Build history of the part. All positions in model axes, mm. A direction names the side the tool comes from. Give positions to 0.01 mm unless a question says otherwise; leave off trailing zeros. Order: outer loops, then holes, each group sorted by start corner. A loop starts at its lowest first (then second) coordinate and runs counter-clockwise, first axis right, second up. Notation, with made-up numbers: (2.25, 50) - (6.25, 50) arc R17 cw to (6.25, 82) - close; hole circle Ø4 at (34, 73). An arc over 180 degrees is marked (long way). Use a Markdown table: item, result.
from build123d import *

# Parameters (mm, degrees)
F0_W     = 3.175
F0_H     = 66.04
F1_DEPTH = 3.175
F2_DEPTH = 66.04
F3_R     = 5.08
F4_W     = 70.348228
F4_H     = 17.78
F5_DEPTH = 3.175
F4_R     = 5.08
F4_R_2   = 3.556
F6_DEPTH = 25.4
F7_R     = 0.508


with BuildPart() as f1:
    # F0 (on Top) → F1 (new body)
    with BuildSketch(Plane.XY):
        with Locations((42.8625, 0)):
            Rectangle(F0_W, F0_H)
        with Locations((-42.8625, 0)):
            Rectangle(F0_W, F0_H)
        with BuildLine():
            Line((41.275, -33.02), (41.275, 33.02))
            Line((41.275, 33.02), (3.81, 33.02))
            ThreePointArc((3.81, 33.02), (0, 29.21), (-3.81, 33.02))
            Line((-3.81, 33.02), (-41.275, 33.02))
            Line((-41.275, 33.02), (-41.275, -33.02))
            Line((-41.275, -33.02), (41.275, -33.02))
        make_face()
    extrude(amount=F1_DEPTH)

    # F0 (on Top) → F2 (join)
    with BuildSketch(Plane.XY):
        with Locations((-42.8625, 0)):
            Rectangle(F0_W, F0_H)
        with Locations((42.8625, 0)):
            Rectangle(F0_W, F0_H)
    extrude(amount=-F2_DEPTH)

    # F3
    f3_edges = [f1.edges().sort_by_distance(p)[0] for p in [
        (-44.45, 0, 3.175),
        (44.45, 0, 3.175),
    ]]
    fillet(f3_edges, radius=F3_R)

    # F4 (on face) → F5 (join)
    with BuildSketch(Plane(origin=(0, 0, 0), x_dir=(1, 0, 0), z_dir=(0, 0, -1))):
        Rectangle(F4_W, F4_H)
        Polygon((-18.800886, 0), (-22.100443, -5.715), (-28.699557, -5.715), (-31.999114, 0), (-28.699557, 5.715), (-22.100443, 5.715), align=None, mode=Mode.SUBTRACT)
        Polygon((30.23935, 0), (27.819675, -4.191), (22.980325, -4.191), (20.56065, 0), (22.980325, 4.191), (27.819675, 4.191), align=None, mode=Mode.SUBTRACT)
    extrude(amount=F5_DEPTH)

    # F4 (on face) → F6 (cut)
    with BuildSketch(Plane(origin=(0, 0, 0), x_dir=(1, 0, 0), z_dir=(0, 0, -1))):
        with Locations((-25.4, 0)):
            Circle(F4_R)
        with Locations((25.4, 0)):
            Circle(F4_R_2)
    extrude(amount=-F6_DEPTH, mode=Mode.SUBTRACT)

    # F7
    f7_edges = [f1.edges().sort_by_distance(p)[0] for p in [
        (35.174114, 0, -3.175),
        (0, -8.89, -3.175),
        (-35.174114, 0, -3.175),
        (0, 8.89, -3.175),
        (-20.450665, 2.8575, -3.175),
        (-25.4, 5.715, -3.175),
        (-30.349335, 2.8575, -3.175),
        (-30.349335, -2.8575, -3.175),
        (-25.4, -5.715, -3.175),
        (-20.450665, -2.8575, -3.175),
        (29.029512, -2.0955, -3.175),
        (29.029512, 2.0955, -3.175),
        (25.4, 4.191, -3.175),
        (21.770488, 2.0955, -3.175),
        (21.770488, -2.0955, -3.175),
        (25.4, -4.191, -3.175),
    ]]
    fillet(f7_edges, radius=F7_R)


solid = f1.part
1) Wall check: line 1 (Y direction, x = -25.4, z = 0.7); line 2 (X direction, y = 22, z = -7.5) (3 decimals); line 3 (Y direction, x = 25.4, z = 1.45). Give the ranges that are in metal, low to high. Write a range as from..to.
Computed:
| item | result |
|---|---|
| line 1 | y = -33.02..-5.08, 5.08..33.02 |
| line 2 | x = -44.45..-41.275, 41.275..44.45 |
| line 3 | y = -33.02..-3.56, 3.56..33.02 |
2) Tool access for faces 4 (the cylindrical face through (21.847, -0.156, 1.565)), 5 (the flat face through (-1, -14, 0)), 6 (the flat face through (0, 0, -3.175)): list every direction of +Z, -Z, +X, -X, +Y, -Y with a clear straight run to the whole face (end or side of a thin tool).
Computed:
| item | result |
|---|---|
| face 4 | +Z, -Z |
| face 5 | -Z |
| face 6 | -Z, +Y, -Y |
3) Slice it at D-D (y = 26). Write the cut outline in (x, z) (3 decimals).
Computed:
| item | result |
|---|---|
| outline | (-44.45, -66.04) - (-41.275, -66.04) - (-41.275, 0) - (41.275, 0) - (41.275, -66.04) - (44.45, -66.04) - (44.45, -1.905) arc R5.08 ccw to (39.37, 3.175) - (-39.37, 3.175) arc R5.08 ccw to (-44.45, -1.905) - close |
4) Slice it at B-B (x = -25.4). Write the cut outline in (y, z) (3 decimals), and give its area (3 significant figures).
Computed:
| item | result |
|---|---|
| outline | (-33.02, 0) - (-8.89, 0) - (-8.89, -2.667) arc R0.508 ccw to (-8.382, -3.175) - (-6.223, -3.175) arc R0.508 ccw to (-5.715, -2.667) - (-5.715, 0) - (-5.08, 0) - (-5.08, 3.175) - (-33.02, 3.175) - close; (5.08, 0) - (5.715, 0) - (5.715, -2.667) arc R0.508 ccw to (6.223, -3.175) - (8.382, -3.175) arc R0.508 ccw to (8.89, -2.667) - (8.89, 0) - (33.02, 0) - (33.02, 3.175) - (5.08, 3.175) - close |
| area | 197 mm² |
5) Slice it at C-C (x = 17). Write the cut outline in (y, z) (3 decimals), and give its area (3 significant figures).
Computed:
| item | result |
|---|---|
| outline | (-33.02, 0) - (-8.89, 0) - (-8.89, -2.667) arc R0.508 ccw to (-8.382, -3.175) - (8.382, -3.175) arc R0.508 ccw to (8.89, -2.667) - (8.89, 0) - (33.02, 0) - (33.02, 3.175) - (-33.02, 3.175) - close |
| area | 266 mm² |
6) Slice it at A-A (z = -21). Write the cut outline in (x, y) (3 decimals), and give its area (3 significant figures).
Computed:
| item | result |
|---|---|
| outline | (-44.45, -33.02) - (-41.275, -33.02) - (-41.275, 33.02) - (-44.45, 33.02) - close; (41.275, -33.02) - (44.45, -33.02) - (44.45, 33.02) - (41.275, 33.02) - close |
| area | 419 mm² |
7) Two-plate mould, pull along Y, no slides. Class faces 1 (the flat face through (-42, 33.02, -21)), 2 (the flat face through (-41.275, 0, -33)), 3 (the cylindrical face through (29.18, -2.14, -3.03)): +Y half, -Y half, draft (parallel to the pull), parting line (faces both ways), or undercut.
Computed:
| item | result |
|---|---|
| face 1 | +Y half |
| face 2 | draft |
| face 3 | undercut |
8) Pin check, flat tips, straight feed: P1, Ø3, axis at x = 25, z = -2, coming from the +Y side; P2, Ø1, axis at x = 2, y = 16.5, coming from the -Z side; P3, Ø5, axis at x = 14, y = -3, coming from the -Z side (3 decimals); P4, Ø10, axis at x = 7, z = -9.5, coming from the +Y side. Stop position of each tip, or through.
Computed:
| item | result |
|---|---|
| P1 | stops at y = 8.89 |
| P2 | stops at z = 0 |
| P3 | stops at z = -3.175 |
| P4 | passes through |
